Input: part model. Units: mm. Frame: model coordinates. Face numbers are marked on the shaded views. A direction names the side the tool comes from. Give positions to 0.01 mm unless a question says otherwise; leave off trailing zeros. Loops run counter-clockwise (first coordinate to the right, second up) from the corner with the lowest first, then second, coordinate; pieces in that order, holes last.
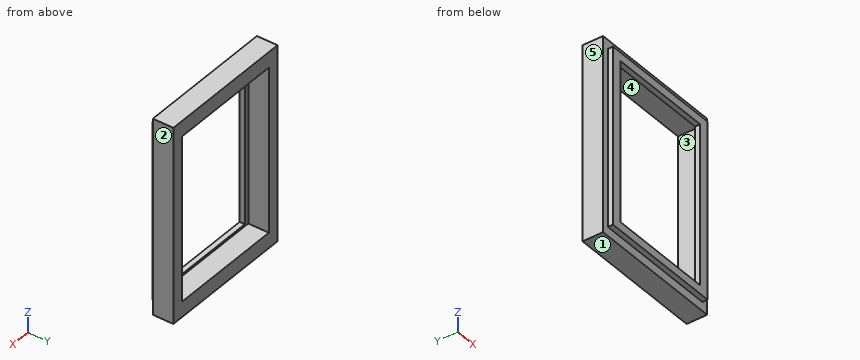
from build123d import *

# Parameters (mm, degrees)
SKETCH3_W           = 108
SKETCH3_H           = 152
BOSS_EXTRUDE1_DEPTH = 16
SKETCH7_W           = 98
SKETCH7_H           = 138
BOSS_EXTRUDE2_DEPTH = 4
SKETCH5_W           = 82.75
SKETCH5_H           = 124.75
CUT_EXTRUDE1_DEPTH  = 96.351979528
SKETCH6_W           = 90
SKETCH6_H           = 128
CUT_EXTRUDE2_DEPTH  = 16


with BuildPart() as part:
    # Sketch3 → Boss-Extrude1 (new body)
    with BuildSketch(Plane(origin=(0, 0, 0), x_dir=(1, 0, 0), z_dir=(0, 1, 0))):
        Rectangle(SKETCH3_W, SKETCH3_H)
    extrude(amount=BOSS_EXTRUDE1_DEPTH)

    # Sketch7 → Boss-Extrude2 (add)
    with BuildSketch(Plane.XZ):
        Rectangle(SKETCH7_W, SKETCH7_H)
    extrude(amount=BOSS_EXTRUDE2_DEPTH)

    # Sketch5 → Cut-Extrude1 (cut, through all)
    with BuildSketch(Plane(origin=(0, 16, 0), x_dir=(1, 0, 0), z_dir=(0, 1, 0))):
        Rectangle(SKETCH5_W, SKETCH5_H)
    extrude(amount=-CUT_EXTRUDE1_DEPTH, mode=Mode.SUBTRACT)

    # Sketch6 → Cut-Extrude2 (cut)
    with BuildSketch(Plane(origin=(0, 16, 0), x_dir=(1, 0, 0), z_dir=(0, 1, 0))):
        Rectangle(SKETCH6_W, SKETCH6_H)
    extrude(amount=-CUT_EXTRUDE2_DEPTH, mode=Mode.SUBTRACT)


solid = part.part
(1) Cut plane C-C (x = 29). Return the cut outline in (y, z) (3 decimals), and give its area (3 significant figures).
Values follow:
outline: (-4, -69) - (0, -69) - (0, -76) - (16, -76) - (16, -64) - (0, -64) - (0, -62.375) - (-4, -62.375) - close; (-4, 62.375) - (0, 62.375) - (0, 64) - (16, 64) - (16, 76) - (0, 76) - (0, 69) - (-4, 69) - close
area: 437 mm2
(2) Pin query (flat end, axial travel): pin 1 Ø1.2 at (x, y) = (-7.5, -2.5) entering from -Z; pin 2 Ø3 at (y, z) = (-3, -26.5) entering from +X; pin 3 Ø3 at (x, y) = (-7, -2.5) entering from +Z. Return the tip coordinate at first contact, or that it passes through.
Values follow:
pin 1: stops at z = -69
pin 2: stops at x = 49
pin 3: stops at z = 69
(3) Cut plane B-B (y = 14.25). Return the cut outline in (x, z).
Values follow:
outline: (-54, -76) - (54, -76) - (54, 76) - (-54, 76) - close; hole (-45, -64) - (45, -64) - (45, 64) - (-45, 64) - close
(4) Ray query, probe 1 along X at (y, z) = (6.75, 33); probe 2 along Z at (x, y) = (43, 14.75); probe 3 along Z at (x, y) = (-21.5, -1.25) (3 decimals). Return the intervals inside material, ascending.
Values follow:
probe 1: x = -54 to -45, 45 to 54
probe 2: z = -76 to -64, 64 to 76
probe 3: z = -69 to -62.375, 62.375 to 69
(5) Mould query, pull axis X, two halves, no side actions, for the marked faces 1, 2 and 3. Classes: +X half, -X half, draft (parallel to the pull), parting line (faces both ways), or undercut.
Values follow:
face 1: draft
face 2: +X half
face 3: undercut
(6) Reachability of the marked faces 4 and 5 from +Z, -Z, +X, -X, +Y, -Y: full face, straight path, thin tool, end or side. Return the list, or none.
Values follow:
face 4: +Y
face 5: +Z, -Z, -X, +Y, -Y
(7) Cut plane A-A (z = 40.5). Return the cut outline in (x, y) (3 decimals).
Values follow:
outline: (-54, 0) - (-49, 0) - (-49, -4) - (-41.375, -4) - (-41.375, 0) - (-45, 0) - (-45, 16) - (-54, 16) - close; (41.375, -4) - (49, -4) - (49, 0) - (54, 0) - (54, 16) - (45, 16) - (45, 0) - (41.375, 0) - close
